Verification items for this drawing (mm, ordinates from the low corner). Give positions to 0.01 mm unless a question says otherwise; leave off trailing zeros. Loops run counter-clockwise (first coordinate to the right, second up) from the corner with the lowest first, then second, coordinate; pieces in that order, holes last. Notation, with made-up numbers: (-13, 64.5) -> (33, 64.5) arc R8 cw to (33, 74.5) -> close; hole circle Ø1 at (19, 9.5). An arc over 180 degrees is marked (long way). Write item = value, one per line.
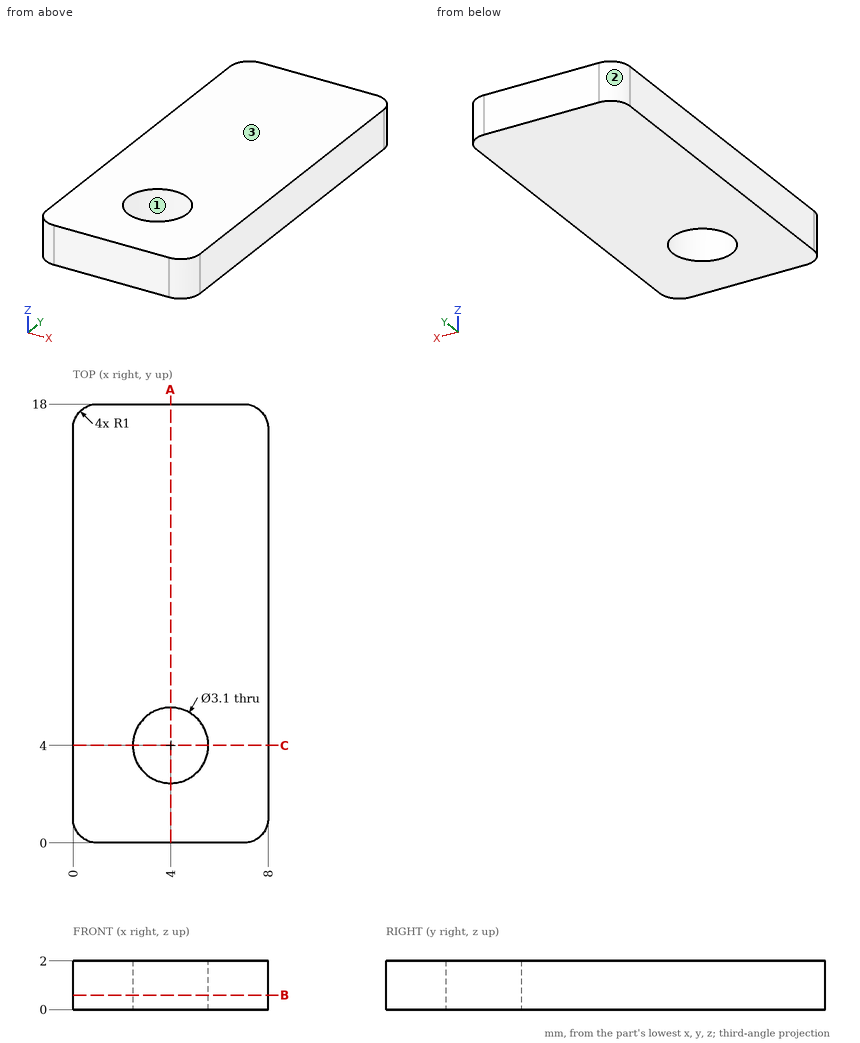
Item 1: Thickness scan on L1, parallel to Y at x = 4, z = 1.1; L2, parallel to X at y = 3.5, z = 1.15; L3, parallel to X at y = 3, z = 0.55. Record the ranges inside material, lowest first. Write a range as [from, to].
Answer:
L1 = [0, 2.45], [5.55, 18]
L2 = [0, 2.53], [5.47, 8]
L3 = [0, 2.82], [5.18, 8]
Item 2: Section check B-B, the plane z = 0.6. Record the cut outline in (x, y), plus the area to 3 significant figures.
Answer:
outline = (0, 1) arc R1 ccw to (1, 0) -> (7, 0) arc R1 ccw to (8, 1) -> (8, 17) arc R1 ccw to (7, 18) -> (1, 18) arc R1 ccw to (0, 17) -> close; hole circle Ø3.1 at (4, 4)
area = 136 mm^2
Item 3: Section check A-A, the plane x = 4. Record the cut outline in (y, z).
Answer:
outline = (0, 0) -> (2.45, 0) -> (2.45, 2) -> (0, 2) -> close; (5.55, 0) -> (18, 0) -> (18, 2) -> (5.55, 2) -> close
Item 4: Gauge pin test, flat end, axial feed: pin 1 (3 mm diameter, centred on x = 4, y = 5.5, fed in from -Z). Record the tip position at first contact, or that the pin passes through.
Answer:
pin_1 = 0
Item 5: Section check C-C, the plane y = 4. Record the cut outline in (x, z), plus the area to 3 significant figures.
Answer:
outline = (0, 0) -> (2.45, 0) -> (2.45, 2) -> (0, 2) -> close; (5.55, 0) -> (8, 0) -> (8, 2) -> (5.55, 2) -> close
area = 9.80 mm^2
Item 6: Draft check along X on the marked faces 1, 2 and 3. Enter one of: +X half, -X half, draft (parallel to the pull), parting line (faces both ways), or undercut.
Answer:
face_1 = undercut
face_2 = -X half
face_3 = draft
